```python
from build123d import *

# Parameters (mm, degrees)
SKETCH_1_R               = 39
EXTRUDE_1_DEPTH          = 4
FILLET_1_R               = 3.5
SKETCH_3_R               = 37
EXTRUDE_2_DEPTH          = 8
SKETCH_4_R               = 36
EXTRUDE_3_DEPTH          = 8
SKETCH_5_W               = 3
SKETCH_5_H               = 1.5
SKETCH_7_R               = 27
CUT_EXTRUDE_1_DEPTH      = 17
CHAMFER_2_SIZE           = 1
SKETCH_18_R              = 1.3
CUT_EXTRUDE_6_DEPTH      = 7
EXTRUDE_START            = 17
SKETCH_19_R              = 27
EXTRUDE_4_DEPTH          = 17
SKETCH_20_R              = 26.5
CUT_EXTRUDE_7_DEPTH      = 15
SKETCH_21_R              = 2.25
CUT_EXTRUDE_8_DEPTH      = 15
SKETCH_23_R              = 1.3
CUT_EXTRUDE_9_DEPTH      = 7
CUT_EXTRUDE_START        = 38
SKETCH_25_R              = 1.5
CUT_EXTRUDE_11_DEPTH     = 4
PATTERN_CIRCULAR_2_COUNT = 2


with BuildPart() as part:
    # Sketch 1 → Бобышка-Вытянуть1 (new body)
    with BuildSketch(Plane.XY):
        Circle(SKETCH_1_R)
    extrude(amount=EXTRUDE_1_DEPTH)

    # Скругление1
    fillet_1_edges = [part.edges().sort_by_distance(p)[0] for p in [
        (-39, 0, 4),
    ]]
    fillet(fillet_1_edges, radius=FILLET_1_R)

    # Эскиз3 → Бобышка-Вытянуть2 (add)
    with BuildSketch(Plane(origin=(0, 0, 0), x_dir=(-1, 0, 0), z_dir=(0, 0, -1))):
        with Locations(Location((0, 0, 0), (0, 0, 180))):
            Circle(SKETCH_3_R)
    extrude(amount=EXTRUDE_2_DEPTH)

    # Эскиз4 → Бобышка-Вытянуть3 (add)
    with BuildSketch(Plane(origin=(0, 0, -8), x_dir=(-1, 0, 0), z_dir=(0, 0, -1))):
        Circle(SKETCH_4_R)
    extrude(amount=EXTRUDE_3_DEPTH)

    # Эскиз5 → Вырез-Повернуть1 (revolve, cut)
    with BuildSketch(Plane(origin=(0, 0, 0), x_dir=(0, 0, -1), z_dir=(1, 0, 0)), mode=Mode.PRIVATE) as cut_revolve_1_sk:
        with Locations((12.5, 35.25)):
            Rectangle(SKETCH_5_W, SKETCH_5_H)
    revolve(cut_revolve_1_sk.sketch.rotate(Axis((0, 0, 46.650977883), (0, 0, -1)), 90), axis=Axis((0, 0, 46.650977883), (0, 0, -1)), mode=Mode.SUBTRACT)

    # Эскиз7 → Вырез-Вытянуть1 (cut)
    with BuildSketch(Plane(origin=(0, 0, -16), x_dir=(-1, 0, 0), z_dir=(0, 0, -1))):
        Circle(SKETCH_7_R)
    extrude(amount=-CUT_EXTRUDE_1_DEPTH, mode=Mode.SUBTRACT)

    # Фаска2
    chamfer_2_edges = [part.edges().sort_by_distance(p)[0] for p in [
        (36, 0, -16),
    ]]
    chamfer(chamfer_2_edges, length=CHAMFER_2_SIZE)

    # Эскиз18 → Вырез-Вытянуть6 (cut)
    with BuildSketch(Plane.XY.offset(4)):
        with Locations((6.5, 32.5)):
            Circle(SKETCH_18_R)
        with Locations(Location((-6.5, 32.5, 0), (0, 0, 180))):
            Circle(SKETCH_18_R)
        with Locations(Location((6.5, -32.5, 0), (0, 0, 180))):
            Circle(SKETCH_18_R)
        with Locations((-6.5, -32.5)):
            Circle(SKETCH_18_R)
    extrude(amount=-CUT_EXTRUDE_6_DEPTH, mode=Mode.SUBTRACT)

    # Эскиз19 → Бобышка-Вытянуть4 (add)
    with BuildSketch(Plane(origin=(0, 0, 1), x_dir=(-1, 0, 0), z_dir=(0, 0, -1)).offset(EXTRUDE_START)):
        Circle(SKETCH_19_R)
    extrude(amount=-EXTRUDE_4_DEPTH)

    # Эскиз20 → Вырез-Вытянуть7 (cut)
    with BuildSketch(Plane.XY.offset(4)):
        Circle(SKETCH_20_R)
    extrude(amount=-CUT_EXTRUDE_7_DEPTH, mode=Mode.SUBTRACT)

    # Эскиз21 → Вырез-Вытянуть8 (cut)
    with BuildSketch(Plane.XY.offset(-11)):
        with Locations((-18, 0)):
            Circle(SKETCH_21_R)
        with Locations((-9, 15.588457268)):
            Circle(SKETCH_21_R)
        with Locations((9, 15.588457268)):
            Circle(SKETCH_21_R)
        with Locations((18, 0)):
            Circle(SKETCH_21_R)
        with Locations((9, -15.588457268)):
            Circle(SKETCH_21_R)
        with Locations((-9, -15.588457268)):
            Circle(SKETCH_21_R)
        Circle(SKETCH_21_R)
    extrude(amount=-CUT_EXTRUDE_8_DEPTH, mode=Mode.SUBTRACT)

    # Эскиз22 → Вырез-Повернуть2 (revolve, cut)
    with BuildSketch(Plane(origin=(0, 0, 0), x_dir=(0, 0, -1), z_dir=(1, 0, 0)), mode=Mode.PRIVATE) as cut_revolve_2_sk:
        Polygon((3.5, 26.5), (5.383390473, 29.817478189), (7.363463637, 26.5), align=None)
    revolve(cut_revolve_2_sk.sketch.rotate(Axis((0, 0, 32.005569053), (0, 0, -1)), 90), axis=Axis((0, 0, 32.005569053), (0, 0, -1)), mode=Mode.SUBTRACT)

    # Эскиз23 → Вырез-Вытянуть9 (cut)
    with BuildSketch(Plane(origin=(0, 0, -16), x_dir=(-1, 0, 0), z_dir=(0, 0, -1))):
        with Locations((23.180408503, 22.060568026)):
            Circle(SKETCH_23_R)
        with Locations(Location((-23.180408503, 22.060568026, 0), (0, 0, 180))):
            Circle(SKETCH_23_R)
        with Locations(Location((23.180408503, -22.060568026, 0), (0, 0, 180))):
            Circle(SKETCH_23_R)
        with Locations((-23.180408503, -22.060568026)):
            Circle(SKETCH_23_R)
    extrude(amount=-CUT_EXTRUDE_9_DEPTH, mode=Mode.SUBTRACT)

    # Эскиз25 → Вырез-Вытянуть11 (cut)
    with BuildSketch(Plane(origin=(0, 0, 0), x_dir=(0, 0, -1), z_dir=(1, 0, 0)).offset(CUT_EXTRUDE_START)):
        with Locations((5, 0)):
            Circle(SKETCH_25_R)
    cut_extrude_11 = extrude(amount=-CUT_EXTRUDE_11_DEPTH, mode=Mode.SUBTRACT)

    # Круговой массив2: Вырез-Вытянуть11 ×2 about axis
    pattern_circular_2_axis = Axis((0, 0, -8), (0, 0, 1))
    for i in range(1, PATTERN_CIRCULAR_2_COUNT):
        add(cut_extrude_11.rotate(pattern_circular_2_axis, i * 360 / PATTERN_CIRCULAR_2_COUNT), mode=Mode.SUBTRACT)


solid = part.part
```
The listing builds one solid part. Answer for the finished solid, in the listing's coordinates (mm). A direction names the side the tool comes from. Coordinates: 2 decimals unless noted, no trailing zeros. Use one line per item in the form item = value. Start each with the question number.
Item 1: A tool of negligible diameter and unlimited length cuts with its end or side. For faces 5 (the face through (-23, 22, -9)), 6 (the face through (-9.488, -17.785, -13.465)), 7 (the face through (7, -33, -3)), from which of +Z, -Z, +X, -X, +Y, -Y can it reach the whole face along a straight path? Write none if from no direction.
Item 2: The part is cut by section A-A on y = 0. Count the separate pieces of the cut face and the enclosed holes in it, then the cut area to 3 significant figures.
Item 3: The mould has two halves that part along Z. Classify faces 1 (the face through (-35.52, -0.45, -6.43)), 2 (the face through (-7, -32, -3)), 3 (the face through (-34, 0, -5)), 4 (the face through (24.42, 21.67, -12.55)): released by +Z, released by -Z, zero draft, split by the parting line, or undercut.
Item 4: Consider L1, parallel to X at y = -1, z = -11.5; L2, parallel to Z at x = 12, y = 22; L3, parallel to Y at x = -4, z = -6. Determine where each line is inside the solid, lowest interval first. Write a range as [from, to].
Item 5: Flat-ended cylindrical pins translate along their axes: pin 1 Ø1 at (x, z) = (-25, -8) entering from -Y; pin 2 Ø1 at (x, z) = (-22, -13) entering from +Y; pin 3 Ø2.5 at (x, y) = (-23.18, 22.06) entering from -Z. Find the tip coordinate at first contact, or state that the pin passes through.
Answer key:
q1.face_5 = -Z
q1.face_6 = +Z, -Z
q1.face_7 = +Z
q2.separate_pieces = 4
q2.enclosed_holes = 0
q2.area = 571 mm2
q3.face_1 = undercut
q3.face_2 = released by +Z
q3.face_3 = undercut
q3.face_4 = zero draft
q4.L1 = [-34.49, -20.02], [-15.98, -2.02], [2.02, 15.98], [20.02, 34.49]
q4.L2 = [-16, -11]
q4.L3 = [-36.78, -28.51], [28.51, 36.78]
q5.pin_1 = -27.73
q5.pin_2 = 26.98
q5.pin_3 = -9
